Print and shaded views of the part. All mm, measured from the part's lowest x, y and z. A direction names the side the tool comes from. Coordinates: 2 decimals unless noted, no trailing zeros. Loops run counter-clockwise (first coordinate to the right, second up) from the corner with the lowest first, then second, coordinate; pieces in that order, holes last. Notation, with made-up numbers: M 67,39 L 96,39 A24 ccw 96,75 Z; hole C 89,35 d7. An arc over 180 degrees is marked long. Answer as a JSON object with one key per item and string values. Group by question number.
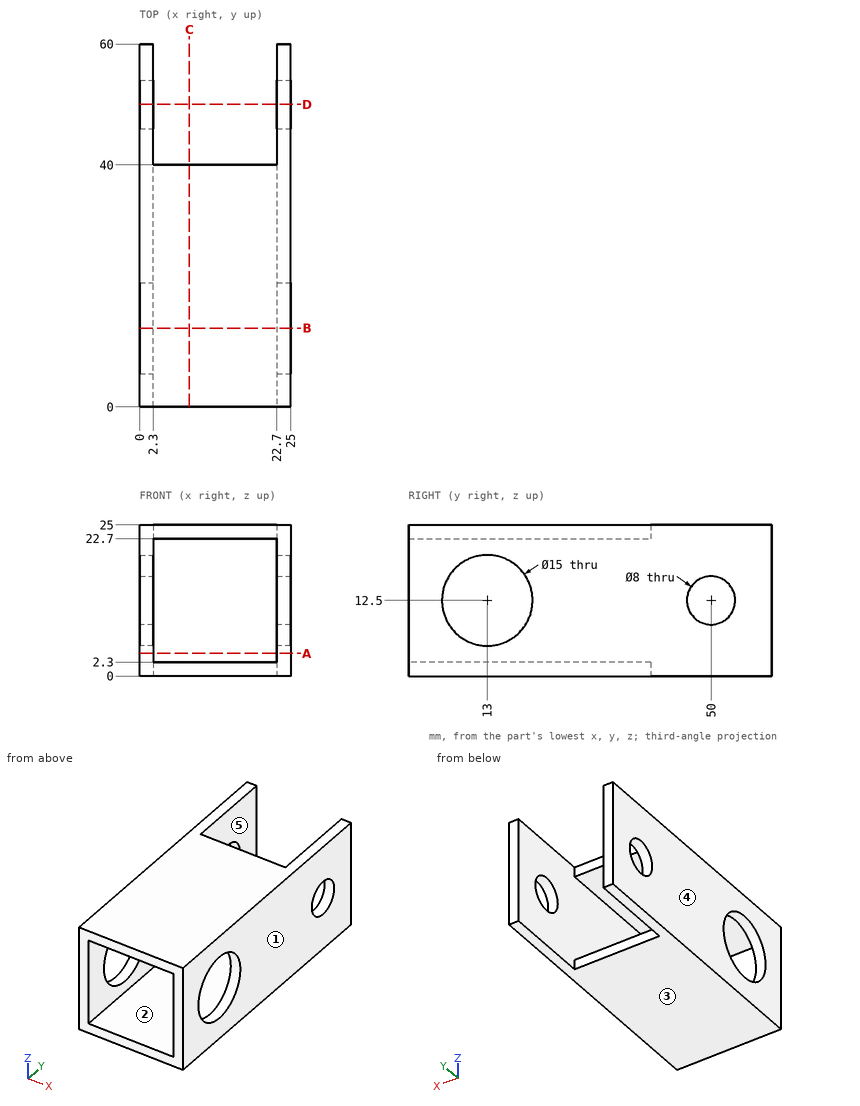
Item 1: Slice it at D-D, the plane y = 50. Write the cut outline in (x, z).
Item 2: Slice it at B-B, the plane y = 13. Write the cut outline in (x, z), then the cut area to 3 significant figures.
Item 3: Slice it at A-A, the plane z = 3.75. Write the cut outline in (x, y), then the cut area to 3 significant figures.
Item 4: Pin check, flat tips, straight feed: pin 1 (0.7 mm diameter, centred on x = 9, z = 23.5, fed in from +Y); pin 2 (6.5 mm diameter, centred on y = 50, z = 12.5, fed in from +X). Stop position of each tip, or through.
Item 5: Drill centre lines: L1, parallel to Y at x = 1.8, z = 12.5; L2, parallel to Z at x = 9, y = 36. Where is each one in solid material? Low to high. Write a range as from..to.
Item 6: Tool access for the marked faces 1 and 2: list every direction of +Z, -Z, +X, -X, +Y, -Y with a clear straight run to the whole face (end or side of a thin tool).
Item 7: Slice it at C-C, the plane x = 8.25. Write the cut outline in (y, z), then the cut area to 3 significant figures.
Item 8: Pull direction Z, two halves, no side cores. Call the marked faces 3, 4 and 5: released by +Z, released by -Z, zero draft, split by the parting line, or undercut.
Computed:
{
 "1": {"outline": "M 0,0 L 2.3,0 L 2.3,8.5 L 0,8.5 Z; M 0,16.5 L 2.3,16.5 L 2.3,25 L 0,25 Z; M 22.7,0 L 25,0 L 25,8.5 L 22.7,8.5 Z; M 22.7,16.5 L 25,16.5 L 25,25 L 22.7,25 Z"},
 "2": {"outline": "M 0,0 L 25,0 L 25,5 L 22.7,5 L 22.7,2.3 L 2.3,2.3 L 2.3,5 L 0,5 Z; M 0,20 L 2.3,20 L 2.3,22.7 L 22.7,22.7 L 22.7,20 L 25,20 L 25,25 L 0,25 Z", "area": "140 mm2"},
 "3": {"outline": "M 0,0 L 2.3,0 L 2.3,60 L 0,60 Z; M 22.7,0 L 25,0 L 25,60 L 22.7,60 Z", "area": "276 mm2"},
 "4": {"pin 1": "y = 40", "pin 2": "through"},
 "5": {"L1": "0..5.5, 20.5..46, 54..60", "L2": "0..2.3, 22.7..25"},
 "6": {"face 1": "+Z, -Z, +X, +Y, -Y", "face 2": "+Y, -Y"},
 "7": {"outline": "M 0,0 L 40,0 L 40,2.3 L 0,2.3 Z; M 0,22.7 L 40,22.7 L 40,25 L 0,25 Z", "area": "184 mm2"},
 "8": {"face 3": "released by -Z", "face 4": "zero draft", "face 5": "undercut"}
}
